from build123d import *

# Parameters (mm, degrees)
CUT_EXTRUDE3_START = -40.72
SKETCH15_R         = 10
CUT_EXTRUDE3_DEPTH = 40.72
SKETCH16_R         = 5
CUT_EXTRUDE4_DEPTH = 40.72


with BuildPart() as part:
    # Sketch1 → Revolve5 (revolve)
    with BuildSketch(Plane.XY, mode=Mode.PRIVATE) as revolve5_sk:
        Polygon((0, 0), (0, 10), (-12, 10), (-12, 16), (0, 18), (0, 35), (-12, 38), (-12, 48), (23, 48), (23, 38), (11, 35), (11, 18), (23, 16), (23, 10), (11, 10), (11, 0), align=None)
    revolve(revolve5_sk.sketch.rotate(Axis((11, 0, 0), (-1, 0, 0)), 90), axis=Axis((11, 0, 0), (-1, 0, 0)))

    # Sketch15 → Cut-Extrude3 (cut)
    with BuildSketch(Plane(origin=(11, 0, 0), x_dir=(0, 0, -1), z_dir=(1, 0, 0)).offset(CUT_EXTRUDE3_START)):
        Circle(SKETCH15_R)
    extrude(amount=CUT_EXTRUDE3_DEPTH, mode=Mode.SUBTRACT)

    # Sketch16 → Cut-Extrude4 (cut)
    with BuildSketch(Plane.ZY.offset(12)):
        with Locations((0, 26.5)):
            Circle(SKETCH16_R)
        with Locations((26.5, 0)):
            Circle(SKETCH16_R)
        with Locations((0, -26.5)):
            Circle(SKETCH16_R)
        with Locations((-26.5, 0)):
            Circle(SKETCH16_R)
    extrude(amount=-CUT_EXTRUDE4_DEPTH, mode=Mode.SUBTRACT)


solid = part.part
Read the model definition and answer for the solid it produces. Units are mm, in the model's axes. Round coordinates to 2 decimals unless told otherwise and drop trailing zeros. Loops run counter-clockwise (first coordinate to the right, second up) from the corner with the lowest first, then second, coordinate; pieces in that order, holes last. Notation, with made-up numbers: (-8, -31.5) - (41, -31.5) arc R22 cw to (41, -21.5) - close; hole circle Ø11 at (3, 36.5). An arc over 180 degrees is marked (long way). One line per question, with ' | ' between items. Start each with the question number.
Q1. Section A-A on y = 0 is taken. Count the separate pieces of the cut face and the enclosed holes in it, plus the area to 3 significant figures.
Q2. Section D-D on x = 16 is taken. Give the vertices of the cut face in (y, z), plus the area to 3 significant figures.
Q3. For a pull along Y with two mould halves and no side action, classify faces 1 (the cylindrical face through (5.745, -14.418, -45.783)), 2 (the flat face through (0, 15, 15)), 3 (the flat face through (-12, -14.45, 35.33)), 4 (the flat face through (11, 15, -15)) as +Y half, -Y half, draft (parallel to the pull), parting line (faces both ways), or undercut.
Q4. Section C-C on x = 9 is taken. Give the vertices of the cut face in (y, z).
Q5. Find the intervals of material crossed by L1, parallel to Y at x = 7.75, z = 0; L2, parallel to X at y = -8, z = -25.5; L3, parallel to Y at x = -5, z = 0, in increasing order.
Q6. Flat-ended cylindrical pins translate along their axes: pin 1 (10 mm diameter, centred on x = 3, z = 9, fed in from -Y); pin 2 (3 mm diameter, centred on x = -6.5, z = 5, fed in from +Y); pin 3 (4 mm diameter, centred on x = 3.5, z = 20.5, fed in from +Y); pin 4 (8 mm diameter, centred on y = 0, z = 26.5, fed in from -X). Find the tip coordinate at first contact, or state that the pin passes through.
Established:
1) separate pieces: 4 | enclosed holes: 0 | area: 1,500 mm²
2) outline: circle Ø96 at (0, 0); circle Ø34.33 at (0, 0); hole circle Ø72.5 at (0, 0); hole circle Ø20 at (0, 0) | area: 3,720 mm²
3) face 1: parting line | face 2: undercut | face 3: draft | face 4: undercut
4) outline: circle Ø96 at (0, 0); hole circle Ø10 at (-26.5, 0); hole circle Ø20 at (0, 0); hole circle Ø10 at (0, -26.5); hole circle Ø10 at (0, 26.5); hole circle Ø10 at (26.5, 0)
5) L1: -48 to -31.5, -21.5 to -10, 10 to 21.5, 31.5 to 48 | L2: 0 to 11 | L3: -48 to -36.25, -17.17 to -10, 10 to 17.17, 36.25 to 48
6) pin 1: y = -47.83 | pin 2: y = 47.87 | pin 3: y = 44.29 | pin 4: through
